Can you work these out from the drawing? Everything is in mm from the part's minimum corner. A direction names the side the tool comes from. Coordinates: 2 decimals unless noted, no trailing zeros. Order: outer loops, then holes, each group sorted by start corner. A loop starts at its lowest first (then second) coordinate and runs counter-clockwise, first axis right, second up. Notation, with made-up numbers: (28.25, 33) - (81.25, 33) arc R31 ccw to (81.25, 65) - close; hole circle Ø3 at (67, 85.25). An arc over 180 degrees is marked (long way). Use a Markdown table: item, result. Add a question column.
(1) We'd pull the mould along X, two halves only. Please class the marked faces 1, 2 and 3: pulls with the +X half, pulls with the -X half, needs draft (parallel to the pull), parting line crosses it, or undercut.
(2) I want a section at C-C (z = 7). List the corners of the cut face in (x, y) for me, and give its area (3 significant figures).
(3) I want a section at D-D (z = 23). List the corners of the cut face in (x, y) for me, and give its area (3 significant figures).
(4) On a 3-axis mill with a long thin cutter (end or side, diameter ignored), from which of +Z, -Z, +X, -X, +Y, -Y can I reach the whole of each face in a straight line? I mean the marked faces 4, 5 and 6. Say none if no direction works.
(5) I want a section at A-A (x = 12.5). List the corners of the cut face in (y, z) for me, and give its area (3 significant figures).
(6) If I drill on L1, parallel to X at y = 12.5, z = 10.5; L2, parallel to X at y = 12.75, z = 19; L3, parallel to Y at x = 12.5, z = 12.25, over which ranges is the centre line in solid material (lowest first)? Write a range as [from, to].
(7) For pin 1 Ø13 at (x, z) = (12, 17) entering from -Y; pin 2 Ø2 at (y, z) = (22, 11) entering from -X; pin 3 Ø2 at (y, z) = (21.5, 3) entering from +X; pin 4 Ø1 at (y, z) = (5.5, 15.5) entering from +X, each with a flat end and sliding along its axis, tell me the tip position at first contact or that it passes through.
(8) I want a section at B-B (y = 12.5). List the corners of the cut face in (x, z) for me.
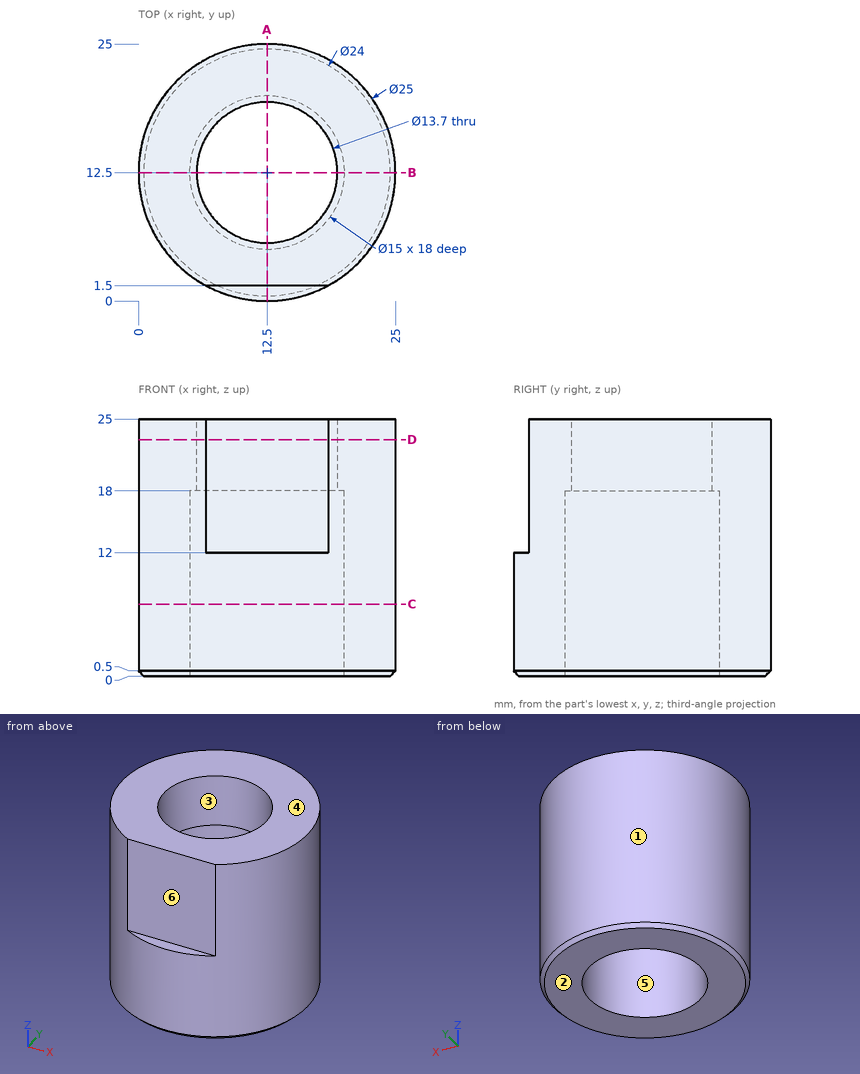
Answers follow:
| question | item | result |
|---|---|---|
| 1 | face 1 | parting line crosses it |
| 1 | face 2 | needs draft |
| 1 | face 3 | undercut |
| 2 | outline | circle Ø25 at (12.5, 12.5); hole circle Ø15 at (12.5, 12.5) |
| 2 | area | 314 mm² |
| 3 | outline | (6.56, 1.5) - (18.44, 1.5) arc R12.5 ccw (long way) to start; hole circle Ø13.7 at (12.5, 12.5) |
| 3 | area | 331 mm² |
| 4 | face 4 | +Z, +X, -X, +Y, -Y |
| 4 | face 5 | -Z |
| 4 | face 6 | +Z, +X, -X, -Y |
| 5 | outline | (0, 0.5) - (0.5, 0) - (5, 0) - (5, 18) - (5.65, 18) - (5.65, 25) - (1.5, 25) - (1.5, 12) - (0, 12) - close; (19.35, 18) - (20, 18) - (20, 0) - (24.5, 0) - (25, 0.5) - (25, 25) - (19.35, 25) - close |
| 5 | area | 239 mm² |
| 6 | L1 | x = [0, 5], [20, 25] |
| 6 | L2 | x = [0, 5.65], [19.35, 25] |
| 6 | L3 | y = [1.5, 5], [20, 25] |
| 7 | pin 1 | stops at y = 0 |
| 7 | pin 2 | stops at x = 3.33 |
| 7 | pin 3 | stops at x = 22.1 |
| 7 | pin 4 | stops at x = 23.18 |
| 8 | outline | (0, 0.5) - (0.5, 0) - (5, 0) - (5, 18) - (5.65, 18) - (5.65, 25) - (0, 25) - close; (19.35, 18) - (20, 18) - (20, 0) - (24.5, 0) - (25, 0.5) - (25, 25) - (19.35, 25) - close |
